The figure shows three views and two pictorial views of one solid part (mm, origin at its lowest corner). Answer the questions. Coordinates: 2 decimals unless noted, no trailing zeros. Loops run counter-clockwise (first coordinate to the right, second up) from the corner with the lowest first, then second, coordinate; pieces in that order, holes last. Notation, with made-up numbers: M 55,17.5 L 69,17.5 A9 ccw 69,27.5 Z; hole C -17,-26 d5. An arc over 180 degrees is marked long. Answer as a JSON object with one key per item and string values. Group by question number.
1. A cutting plane is placed at D-D on z = 145. Give the vertices of the cut face in (x, y), and give its area (3 significant figures).
2. Determine the mould class of the marked faces 1, 2 and 3 for opening direction X: released by +X, released by -X, zero draft, split by the parting line, or undercut.
3. A cutting plane is placed at C-C on z = 105.5. Give the vertices of the cut face in (x, y), and give its area (3 significant figures).
4. A cutting plane is placed at B-B on x = 114. Give the vertices of the cut face in (y, z), and give its area (3 significant figures).
5. Straight lines are drawn through the part: L1, parallel to Y at x = 69.5, z = 56; L2, parallel to X at y = 16, z = 124.5; L3, parallel to X at y = 15.75, z = 101.5. For each, find the intervals that lie inside material, in ascending order.
6. A cutting plane is placed at A-A on y = 14.75. Give the vertices of the cut face in (x, z).
7. Given pin 1 (3 mm diameter, centred on x = 54, z = 31.5, fed in from +Y), flat-ended and moving along its own axis, determine where the tip first touches the part or whether it passes through.
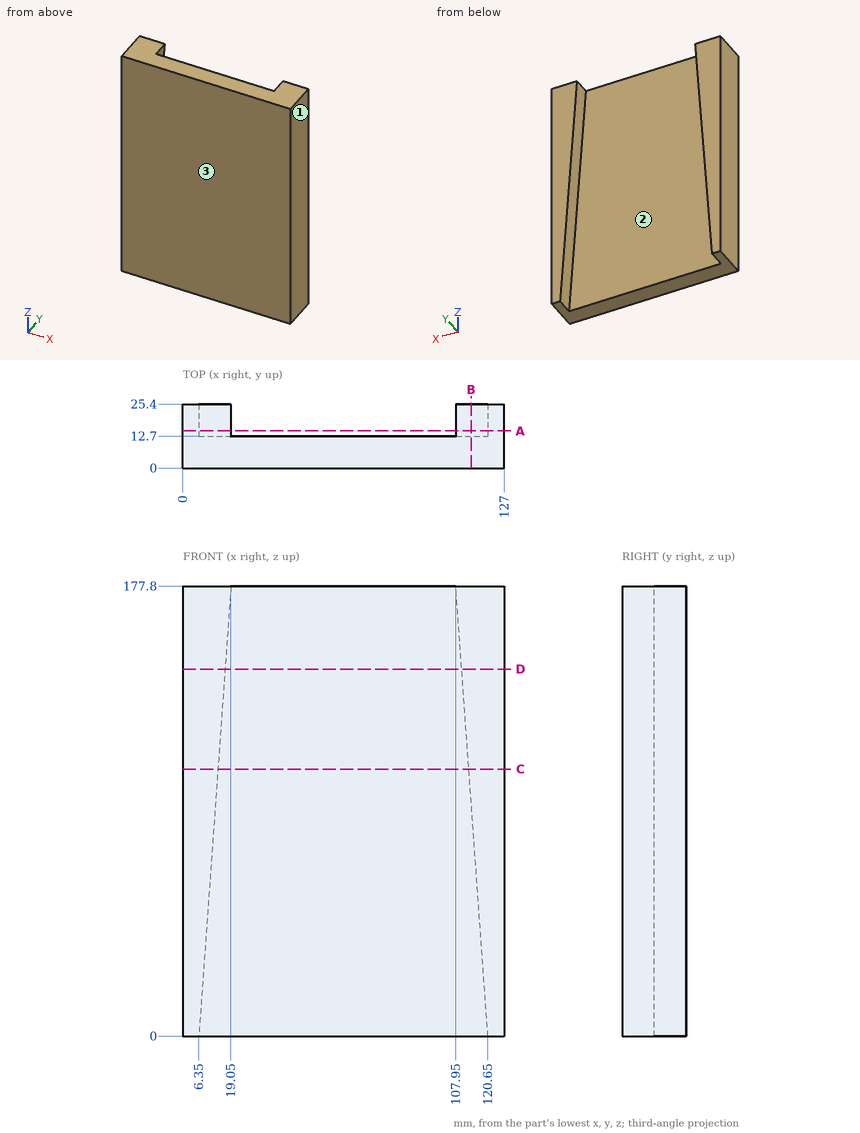
From the geometry:
{
 "1": {"outline": "M 0,0 L 127,0 L 127,25.4 L 110.29,25.4 L 110.29,12.7 L 16.71,12.7 L 16.71,25.4 L 0,25.4 Z", "area": "2,040 mm²"},
 "2": {"face 1": "released by +X", "face 2": "undercut", "face 3": "zero draft"},
 "3": {"outline": "M 0,0 L 127,0 L 127,25.4 L 113.11,25.4 L 113.11,12.7 L 13.89,12.7 L 13.89,25.4 L 0,25.4 Z", "area": "1,970 mm²"},
 "4": {"outline": "M 0,0 L 12.7,0 L 12.7,93.1 L 25.4,93.1 L 25.4,177.8 L 0,177.8 Z", "area": "3,330 mm²"},
 "5": {"L1": "y = 0 to 12.7", "L2": "x = 0 to 15.24, 111.76 to 127", "L3": "x = 0 to 13.6, 113.4 to 127"},
 "6": {"outline": "M 0,0 L 6.35,0 L 19.05,177.8 L 0,177.8 Z; M 107.95,177.8 L 120.65,0 L 127,0 L 127,177.8 Z"},
 "7": {"pin 1": "stops at y = 12.7"}
}
